Here's the drawing with two shaded views (mm, measured from the low corner). I have some questions. Give positions to 0.01 mm unless a question says otherwise; leave off trailing zeros. Write each loop counter-clockwise with the first axis right and the second up, starting at its lowest first coordinate (ties: lowest second). Pieces come first, ordered by that corner, then holes.
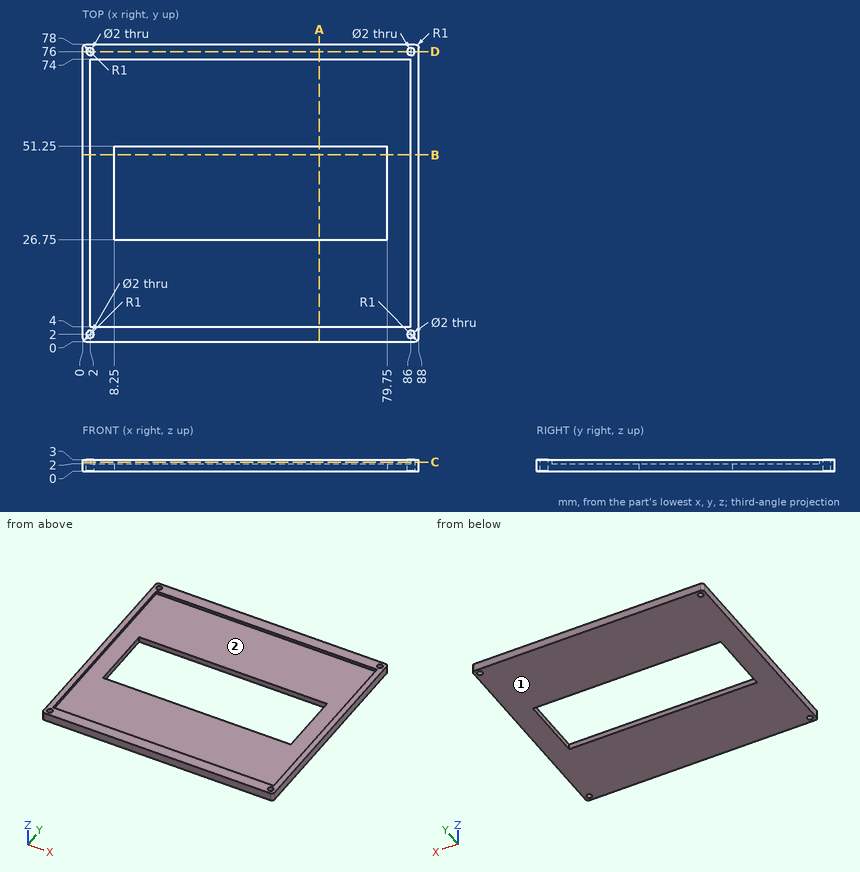
(1) Imagine slicing it at A-A, the plane x = 62. Write out the boundary of the cut face in (y, z).
Returned:
outline: (0, 0) - (26.75, 0) - (26.75, 2) - (4, 2) - (4, 3) - (0, 3) - close; (51.25, 0) - (78, 0) - (78, 3) - (74, 3) - (74, 2) - (51.25, 2) - close
(2) Imagine slicing it at B-B, the plane y = 49. Write out the boundary of the cut face in (x, z), plus the area to 3 significant figures.
Returned:
outline: (0, 0) - (8.25, 0) - (8.25, 2) - (2, 2) - (2, 3) - (0, 3) - close; (79.75, 0) - (88, 0) - (88, 3) - (86, 3) - (86, 2) - (79.75, 2) - close
area: 37.0 mm2
(3) Imagine slicing it at C-C, the plane z = 2.45. Write out the boundary of the cut face in (x, y), plus the area to 3 significant figures.
Returned:
outline: (0, 1) arc R1 ccw to (1, 0) - (87, 0) arc R1 ccw to (88, 1) - (88, 77) arc R1 ccw to (87, 78) - (1, 78) arc R1 ccw to (0, 77) - close; hole circle Ø2 at (2, 2); hole circle Ø2 at (2, 76); hole (2, 4) - (86, 4) - (86, 74) - (2, 74) - close; hole circle Ø2 at (86, 2); hole circle Ø2 at (86, 76)
area: 971 mm2
(4) If we mould it in two halves opening along X, with no side actions, what happens to the marked faces 1 and 2? For each: +X half, -X half, draft (parallel to the pull), parting line (faces both ways), or undercut.
Returned:
face 1: draft
face 2: undercut
(5) If I drill on L1, parallel to Y at x = 86, z = 1.3; L2, parallel to X at y = 76, z = 1.2; L3, parallel to Y at x = 32, z = 2.35, over which ranges is the centre line in solid material (lowest first)?
Returned:
L1: y = 0 to 1, 3 to 75, 77 to 78
L2: x = 0 to 1, 3 to 85, 87 to 88
L3: y = 0 to 4, 74 to 78
(6) Imagine slicing it at D-D, the plane y = 76. Write out the boundary of the cut face in (x, z), plus the area to 3 significant figures.
Returned:
outline: (0, 0) - (1, 0) - (1, 3) - (0, 3) - close; (3, 0) - (85, 0) - (85, 3) - (3, 3) - close; (87, 0) - (88, 0) - (88, 3) - (87, 3) - close
area: 252 mm2
